Build history of the part. All positions in model axes, mm. Give positions to 0.01 mm unless a question says otherwise; leave off trailing zeros. Order: outer loops, then holes, each group sorted by start corner. A loop starts at its lowest first (then second) coordinate and runs counter-clockwise, first axis right, second up. Notation, with made-up numbers: M 47.5,59.25 L 85.5,59.25 A12 cw 85.5,80.25 Z; hole C 21,84 d3. An arc over 180 degrees is marked long. One line per item, written item: value.
from build123d import *

# Parameters (mm, degrees)
SKETCH1_W                                    = 208.28
SKETCH1_H                                    = 266.7
BOSS_EXTRUDE1_DEPTH                          = 4.064
SKETCH2_W                                    = 12.7
SKETCH2_H                                    = 38.1
CUT_EXTRUDE1_DEPTH                           = 170.24502414
FILLET1_R                                    = 3.175
SKETCH3_R                                    = 10
CUT_EXTRUDE2_DEPTH                           = 170.24502414
CSK_FOR_10_FLAT_HEAD_MACHINE_SCREW2_AT_COUNT = 2
CSK_FOR_10_FLAT_HEAD_MACHINE_SCREW2_AT_PITCH = 220.98
CSK_FOR_10_FLAT_HEAD_MACHINE_SCREW2_2_COUNT  = 2
CSK_FOR_10_FLAT_HEAD_MACHINE_SCREW2_2_PITCH  = 176.784
CSK_FOR_10_FLAT_HEAD_MACHINE_SCREW2_3_COUNT  = 2
CSK_FOR_10_FLAT_HEAD_MACHINE_SCREW2_3_PITCH  = 132.588
CSK_FOR_10_FLAT_HEAD_MACHINE_SCREW2_4_COUNT  = 2
CSK_FOR_10_FLAT_HEAD_MACHINE_SCREW2_4_PITCH  = 88.392
CSK_FOR_10_FLAT_HEAD_MACHINE_SCREW2_5_COUNT  = 2
CSK_FOR_10_FLAT_HEAD_MACHINE_SCREW2_5_PITCH  = 44.196


with BuildPart() as part:
    # Sketch1 → Boss-Extrude1 (new body)
    with BuildSketch(Plane(origin=(0, 0, 0), x_dir=(1, 0, 0), z_dir=(0, 1, 0))):
        Rectangle(SKETCH1_W, SKETCH1_H)
    extrude(amount=BOSS_EXTRUDE1_DEPTH)

    # Sketch2 → Cut-Extrude1 (cut, through all)
    with BuildSketch(Plane(origin=(0, 4.064, 0), x_dir=(1, 0, 0), z_dir=(0, 1, 0))):
        with Locations((-53.2265001, 0)):
            Rectangle(SKETCH2_W, SKETCH2_H)
    cut_extrude1 = extrude(amount=-CUT_EXTRUDE1_DEPTH, mode=Mode.SUBTRACT)

    # Mirror1: Cut-Extrude1 across plane
    add(cut_extrude1.mirror(Plane(origin=(0, 0, 0), x_dir=(0, 0, 1), z_dir=(1, 0, 0))), mode=Mode.SUBTRACT)

    # Fillet1
    fillet1_edges = [part.edges().sort_by_distance(p)[0] for p in [
        (-46.8765001, 2.032, -19.05),
        (-46.8765001, 2.032, 19.05),
        (-59.5765001, 2.032, 19.05),
        (-59.5765001, 2.032, -19.05),
        (46.8765001, 2.032, 19.05),
        (46.8765001, 2.032, -19.05),
        (59.5765001, 2.032, -19.05),
        (59.5765001, 2.032, 19.05),
    ]]
    fillet(fillet1_edges, radius=FILLET1_R)

    # Sketch3 → Cut-Extrude2 (cut, through all)
    with BuildSketch(Plane(origin=(0, 0, 0), x_dir=(1, 0, 0), z_dir=(0, 1, 0))):
        with Locations(Location((-89.74, 88.392, 0), (0, 0, 270))):
            Circle(SKETCH3_R)
        with Locations(Location((-89.74, 44.196, 0), (0, 0, 270))):
            Circle(SKETCH3_R)
        with Locations(Location((-89.74, 0, 0), (0, 0, 270))):
            Circle(SKETCH3_R)
        with Locations(Location((-89.74, -44.196, 0), (0, 0, 270))):
            Circle(SKETCH3_R)
        with Locations(Location((-89.74, -88.392, 0), (0, 0, 270))):
            Circle(SKETCH3_R)
    cut_extrude2 = extrude(amount=CUT_EXTRUDE2_DEPTH, mode=Mode.SUBTRACT)

    # Sketch10 → CSK for #10 Flat Head Machine Screw2 (revolve, cut)
    with BuildSketch(Plane(origin=(-91.44, 0, -110.49), x_dir=(0, 0, -1), z_dir=(1, 0, 0))):
        Polygon((0, 0), (0, 12.417662253), (2.4892, 10.922), (2.4892, 2.761229288), (4.8895, 0), align=None)
    csk_for_10_flat_head_machine_screw2 = revolve(axis=Axis((-91.44, -6.35, -110.49), (0, 1, 0)), mode=Mode.SUBTRACT)

    # CSK for #10 Flat Head Machine Screw2 at: CSK for #10 Flat Head Machine Screw2 ×2
    with Locations(*[(0, 0, i * CSK_FOR_10_FLAT_HEAD_MACHINE_SCREW2_AT_PITCH) for i in range(1, CSK_FOR_10_FLAT_HEAD_MACHINE_SCREW2_AT_COUNT)]):
        add(csk_for_10_flat_head_machine_screw2, mode=Mode.SUBTRACT)

    # CSK for _10 Flat Head Machine Screw2 2: CSK for #10 Flat Head Machine Screw2 ×2
    with Locations(*[(0, 0, i * CSK_FOR_10_FLAT_HEAD_MACHINE_SCREW2_2_PITCH) for i in range(1, CSK_FOR_10_FLAT_HEAD_MACHINE_SCREW2_2_COUNT)]):
        add(csk_for_10_flat_head_machine_screw2, mode=Mode.SUBTRACT)

    # CSK for _10 Flat Head Machine Screw2 3: CSK for #10 Flat Head Machine Screw2 ×2
    with Locations(*[(0, 0, i * CSK_FOR_10_FLAT_HEAD_MACHINE_SCREW2_3_PITCH) for i in range(1, CSK_FOR_10_FLAT_HEAD_MACHINE_SCREW2_3_COUNT)]):
        add(csk_for_10_flat_head_machine_screw2, mode=Mode.SUBTRACT)

    # CSK for _10 Flat Head Machine Screw2 4: CSK for #10 Flat Head Machine Screw2 ×2
    with Locations(*[(0, 0, i * CSK_FOR_10_FLAT_HEAD_MACHINE_SCREW2_4_PITCH) for i in range(1, CSK_FOR_10_FLAT_HEAD_MACHINE_SCREW2_4_COUNT)]):
        add(csk_for_10_flat_head_machine_screw2, mode=Mode.SUBTRACT)

    # CSK for _10 Flat Head Machine Screw2 5: CSK for #10 Flat Head Machine Screw2 ×2
    with Locations(*[(0, 0, i * CSK_FOR_10_FLAT_HEAD_MACHINE_SCREW2_5_PITCH) for i in range(1, CSK_FOR_10_FLAT_HEAD_MACHINE_SCREW2_5_COUNT)]):
        add(csk_for_10_flat_head_machine_screw2, mode=Mode.SUBTRACT)

    # Mirror2: Cut-Extrude2, CSK for #10 Flat Head Machine Screw2 across plane
    add(cut_extrude2.mirror(Plane(origin=(0, 0, 0), x_dir=(0, 0, 1), z_dir=(1, 0, 0))), mode=Mode.SUBTRACT)
    add(csk_for_10_flat_head_machine_screw2.mirror(Plane(origin=(0, 0, 0), x_dir=(0, 0, 1), z_dir=(1, 0, 0))), mode=Mode.SUBTRACT)

    # Mirror2 copy 1 sketch → Mirror2 copy 1 (revolve, cut)
    with BuildSketch(Plane(origin=(91.44, 0, 110.49), x_dir=(0, 0, -1), z_dir=(-1, 0, 0))):
        Polygon((0, 0), (0, -12.417662253), (2.4892, -10.922), (2.4892, -2.761229288), (4.8895, 0), align=None)
    revolve(axis=Axis((91.44, -6.35, 110.49), (0, -1, 0)), mode=Mode.SUBTRACT)

    # Mirror2 copy 2 sketch → Mirror2 copy 2 (revolve, cut)
    with BuildSketch(Plane(origin=(91.44, 0, 66.294), x_dir=(0, 0, -1), z_dir=(-1, 0, 0))):
        Polygon((0, 0), (0, -12.417662253), (2.4892, -10.922), (2.4892, -2.761229288), (4.8895, 0), align=None)
    revolve(axis=Axis((91.44, -6.35, 66.294), (0, -1, 0)), mode=Mode.SUBTRACT)

    # Mirror2 copy 3 sketch → Mirror2 copy 3 (revolve, cut)
    with BuildSketch(Plane(origin=(91.44, 0, 22.098), x_dir=(0, 0, -1), z_dir=(-1, 0, 0))):
        Polygon((0, 0), (0, -12.417662253), (2.4892, -10.922), (2.4892, -2.761229288), (4.8895, 0), align=None)
    revolve(axis=Axis((91.44, -6.35, 22.098), (0, -1, 0)), mode=Mode.SUBTRACT)

    # Mirror2 copy 4 sketch → Mirror2 copy 4 (revolve, cut)
    with BuildSketch(Plane(origin=(91.44, 0, -22.098), x_dir=(0, 0, -1), z_dir=(-1, 0, 0))):
        Polygon((0, 0), (0, -12.417662253), (2.4892, -10.922), (2.4892, -2.761229288), (4.8895, 0), align=None)
    revolve(axis=Axis((91.44, -6.35, -22.098), (0, -1, 0)), mode=Mode.SUBTRACT)

    # Mirror2 copy 5 sketch → Mirror2 copy 5 (revolve, cut)
    with BuildSketch(Plane(origin=(91.44, 0, -66.294), x_dir=(0, 0, -1), z_dir=(-1, 0, 0))):
        Polygon((0, 0), (0, -12.417662253), (2.4892, -10.922), (2.4892, -2.761229288), (4.8895, 0), align=None)
    revolve(axis=Axis((91.44, -6.35, -66.294), (0, -1, 0)), mode=Mode.SUBTRACT)


solid = part.part
1) Pin check, flat tips, straight feed: pin 1 (6.5 mm diameter, centred on x = -91.44, z = 22.098, fed in from -Y); pin 2 (3 mm diameter, centred on x = 91.44, z = 110.49, fed in from +Y). Stop position of each tip, or through.
Check values:
pin 1: y = 1.89
pin 2: through
2) Saw through at A-A, the plane z = 0. Write the cut outline in (x, y), then the cut area to 3 significant figures.
Check values:
outline: M -104.14,0 L -99.74,0 L -99.74,4.06 L -104.14,4.06 Z; M -79.74,0 L -59.58,0 L -59.58,4.06 L -79.74,4.06 Z; M -46.88,0 L 46.88,0 L 46.88,4.06 L -46.88,4.06 Z; M 59.58,0 L 79.74,0 L 79.74,4.06 L 59.58,4.06 Z; M 99.74,0 L 104.14,0 L 104.14,4.06 L 99.74,4.06 Z
area: 581 mm^2
3) Drill centre lines: probe 1 along X at (y, z) = (3.55, 110.49); probe 2 along X at (y, z) = (1.85, 13); probe 3 along X at (y, z) = (2.9, 0). Where is each one in solid material? Low to high. Write a range as from..to.
Check values:
probe 1: -104.14..-93.93, -88.95..88.95, 93.93..104.14
probe 2: -104.14..-59.58, -46.88..46.88, 59.58..104.14
probe 3: -104.14..-99.74, -79.74..-59.58, -46.88..46.88, 59.58..79.74, 99.74..104.14
4) Mould opens along Z. For faces 1 (the face through (99.5, 2, -2.17)), 2 (the face through (-1, 4.064, -2)), 3 (the face through (-94.057, 2.588, -110.146)) say: released by +Z, released by -Z, zero draft, split by the parting line, or undercut.
Check values:
face 1: undercut
face 2: zero draft
face 3: undercut
5) Saw through at B-B, the plane y = 1.8. Give the number of separate pieces and of enclosed holes in the cut face, then the cut area to 3 significant figures.
Check values:
separate pieces: 1
enclosed holes: 24
area: 51,000 mm^2
